```python
from build123d import *

# Parameters (mm, degrees)
SKETCH_W        = 120
SKETCH_H        = 120
PAD_DEPTH       = 20
SKETCH001_R     = 4.75
POCKET_DEPTH    = 20.001
SKETCH002_R     = 11
POCKET001_DEPTH = 3


with BuildPart() as part:
    # Sketch → Pad (new body)
    with BuildSketch(Plane.XY):
        Rectangle(SKETCH_W, SKETCH_H)
    extrude(amount=PAD_DEPTH)

    # Sketch001 (on Face6 of Pad) → Pocket (cut, through all)
    with BuildSketch(Plane.XY.offset(20)):
        Circle(SKETCH001_R)
    extrude(amount=-POCKET_DEPTH, mode=Mode.SUBTRACT)

    # Sketch002 (on Face5 of Pocket) → Pocket001 (cut)
    with BuildSketch(Plane.XY.offset(20)):
        Circle(SKETCH002_R)
    extrude(amount=-POCKET001_DEPTH, mode=Mode.SUBTRACT)


solid = part.part
```
Here's how the part is built. I have some questions about the finished solid (model axes, mm). A direction names the side the tool comes from. Round coordinates to 2 decimals unless told otherwise and drop trailing zeros. Write each loop counter-clockwise with the first axis right and the second up, starting at its lowest first coordinate (ties: lowest second). Pieces come first, ordered by that corner, then holes.
Q1. Which directions (+Z, -Z, +X, -X, +Y, -Y) give clear straight access to the entire face, cutting with the end or side of a thin tool? Please do faces 1 (the flat face through (-1, -60, 10)), 2 (the flat face through (2, -5, 17)).
Q2. If we section it at A-A on x = 0: Write out the boundary of the cut face in (y, z).
Q3. If we mould it in two halves opening along X, with no side actions, what happens to faces 3 (the flat face through (60, -1, 10)), 4 (the cylindrical face through (-2.38, -10.74, 18.52)), 5 (the flat face through (-14, 1, 20))? For each: +X half, -X half, draft (parallel to the pull), parting line (faces both ways), or undercut.
Q4. Please list where these lines run through material, in increasing order: probe 1 along Y at (x, z) = (0, 6.5); probe 2 along Y at (x, z) = (0, 18.4); probe 3 along X at (y, z) = (-1.5, 9.25).
Answer below:
1. face 1: +Z, -Z, +X, -X, -Y
1. face 2: +Z
2. outline: (-60, 0) - (-4.75, 0) - (-4.75, 17) - (-11, 17) - (-11, 20) - (-60, 20) - close; (4.75, 0) - (60, 0) - (60, 20) - (11, 20) - (11, 17) - (4.75, 17) - close
3. face 3: +X half
3. face 4: undercut
3. face 5: draft
4. probe 1: y = -60 to -4.75, 4.75 to 60
4. probe 2: y = -60 to -11, 11 to 60
4. probe 3: x = -60 to -4.51, 4.51 to 60
